Verification items for this drawing (mm, ordinates from the low corner). Coordinates: 2 decimals unless noted, no trailing zeros. Order: outer loops, then holes, each group sorted by start corner. A loop starts at its lowest first (then second) coordinate and runs counter-clockwise, first axis right, second up. Notation, with made-up numbers: (20.5, 62) -> (45.5, 62) arc R20 ccw to (45.5, 92) -> close; hole circle Ø8 at (26, 89). An arc over 180 degrees is marked (long way). Answer in a Markdown table with one row per item. Add a question column.
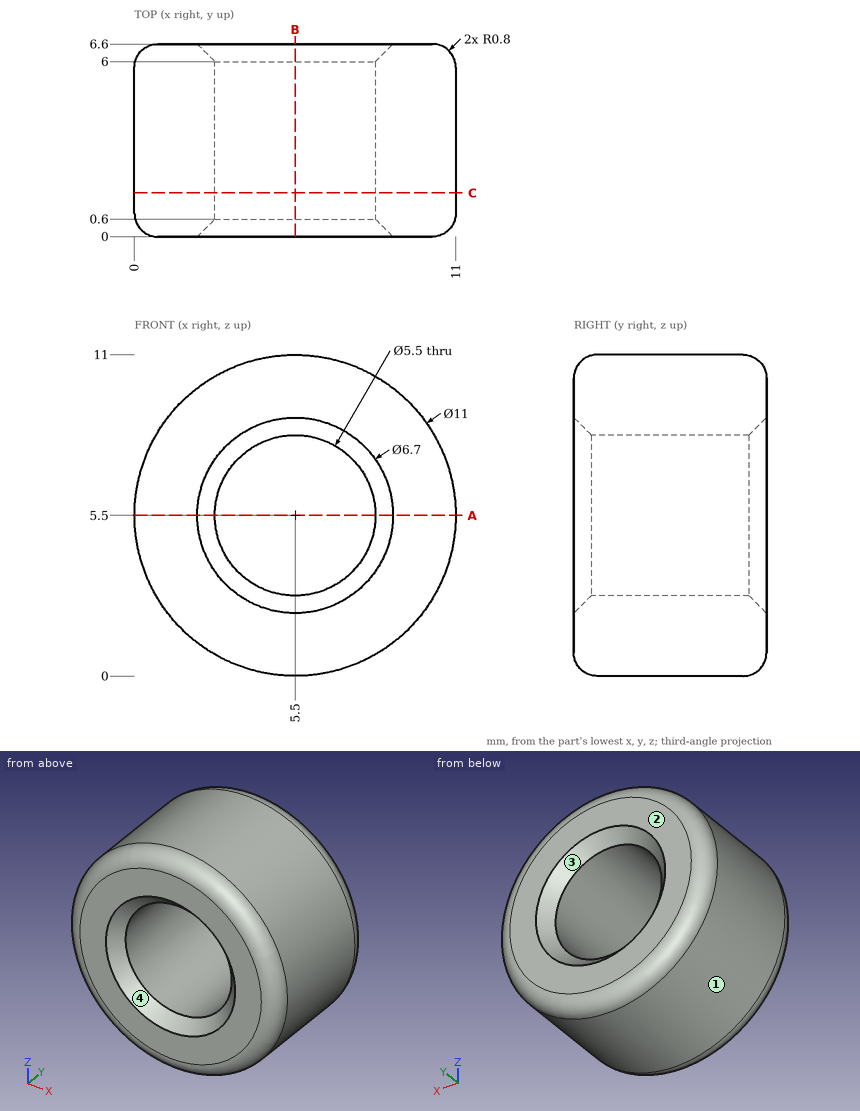
(1) Go/stop test with flat-tipped pins: P1, Ø2, axis at y = 5.5, z = 3.5, coming from the -X side; P2, Ø1, axis at y = 3.5, z = 7.5, coming from the +X side; P3, Ø3, axis at x = 10, y = 2.5, coming from the -Z side; P4, Ø2, axis at x = 4.5, y = 3, coming from the -Z side. Record where each tip stops, or that it passes through.
(2) Mould release check, pull along Z, two halves, no side actions. Record for the marked faces 1, 2, 3 and 4: +Z half, -Z half, draft (parallel to the pull), parting line (faces both ways), or undercut.
(3) Scan lines: line 1 along Z through (x, y) = (5.5, 3.9); line 2 along X through (y, z) = (1.5, 7); line 3 along X through (y, z) = (5.25, 7.75). Record each from-to range of solid material in increasing order.
(4) Cross-section at C-C (y = 1.5). Enter the section's corners in (x, z).
(5) Cross-section at B-B (x = 5.5). Enter the section's corners in (y, z), plus the area to 3 significant figures.
(6) Cross-section at A-A (z = 5.5). Enter the section's corners in (x, y).
Checks:
| question | item | result |
|---|---|---|
| 1 | P1 | x = 0.09 |
| 1 | P2 | x = 10.79 |
| 1 | P3 | z = 0.89 |
| 1 | P4 | z = 0 |
| 2 | face 1 | parting line |
| 2 | face 2 | draft |
| 2 | face 3 | undercut |
| 2 | face 4 | undercut |
| 3 | line 1 | 0 to 2.75, 8.25 to 11 |
| 3 | line 2 | 0.21 to 3.2, 7.8 to 10.79 |
| 3 | line 3 | 0.48 to 3.92, 7.08 to 10.52 |
| 4 | outline | circle Ø11 at (5.5, 5.5); hole circle Ø5.5 at (5.5, 5.5) |
| 5 | outline | (0, 0.8) arc R0.8 ccw to (0.8, 0) -> (5.8, 0) arc R0.8 ccw to (6.6, 0.8) -> (6.6, 2.15) -> (6, 2.75) -> (0.6, 2.75) -> (0, 2.15) -> close; (0, 8.85) -> (0.6, 8.25) -> (6, 8.25) -> (6.6, 8.85) -> (6.6, 10.2) arc R0.8 ccw to (5.8, 11) -> (0.8, 11) arc R0.8 ccw to (0, 10.2) -> close |
| 5 | area | 35.0 mm² |
| 6 | outline | (0, 0.8) arc R0.8 ccw to (0.8, 0) -> (2.15, 0) -> (2.75, 0.6) -> (2.75, 6) -> (2.15, 6.6) -> (0.8, 6.6) arc R0.8 ccw to (0, 5.8) -> close; (8.25, 0.6) -> (8.85, 0) -> (10.2, 0) arc R0.8 ccw to (11, 0.8) -> (11, 5.8) arc R0.8 ccw to (10.2, 6.6) -> (8.85, 6.6) -> (8.25, 6) -> close |
